Input: part model. Units: mm. Frame: model coordinates. A direction names the side the tool comes from. Coordinates: 2 decimals unless noted, no trailing zeros. Write each loop counter-clockwise with the first axis right and the second up, starting at its lowest first coordinate (ties: lowest second). Pieces come first, ordered by that corner, then holes. Notation, with made-up numbers: M 57.25,89 L 109.25,89 A20 cw 109.25,110 Z; hole C -33.5,56.25 d5. An arc over 180 degrees is marked long. Use CSV: the item, a comma, the result in double quotes.
Autodesk Inventor part; units mm, degrees
ref_plane "YZ Plane" through (0, 0, 0) normal (1, 0, 0) x (0, 1, 0)
ref_plane "XZ Plane" through (0, 0, 0) normal (0, 1, 0) x (-1, 0, 0)
ref_plane "XY Plane" through (0, 0, 0) normal (0, 0, 1) x (1, 0, 0)
sketch "Sketch1" plane through (0, 0, 0) normal (0, 1, 0) x (-1, 0, 0)
  circle A0 centre (0, 0) radius 10 construction
  circle A1 centre (0, 0) radius 16
  circle A2 centre (0, 0) radius 11
  circle A3 centre (0, 0) radius 9
  dimension "d0" = 20
  dimension "d1" = 6
  dimension "d4" = 1
  dimension "d9" = 2
extrude "Extrusion1" add sketch "Sketch1" along normal blind 2 contours A1 | A2 | A3
extrude "Extrusion2" add sketch "Sketch1" against normal blind 3 contours A2 | A3
extrude "Extrusion4" cut sketch "Sketch1" along normal through all both and the other way through all contours A3
sketch "Sketch4" plane through (0, 2, 0) normal (0, 1, 0) x (1, 0, 0)
  circle A0 centre (0, 0) radius 16
  line L0 (16, -14.5) -> (-16, -14.5)
  line L1 (-16, -14.5) -> (-16, 14.5)
  line L2 (-16, 14.5) -> (16, 14.5)
  line L3 (16, 14.5) -> (16, -14.5)
  line L4 (16, -14.5) -> (-16, 14.5) construction
  line L5 (-16, -14.5) -> (16, 14.5) construction
  line L6 (-17.5, -16) -> (17.5, -16)
  line L7 (17.5, -16) -> (17.5, 16)
  line L8 (17.5, 16) -> (-17.5, 16)
  line L9 (-17.5, 16) -> (-17.5, -16)
  dimension "d18" = 29
extrude "Extrusion6" cut sketch "Sketch4" against normal up to surface (2 mm away) contours L3 L2 A0 L8 L7 L6 L0 | L2 A0 | A0 L0 | A0 L2 L1 L0 L6 L9 L8
fillet "Fillet1" radius 5 4 edges at (-6.7639, 1, 14.5) (6.7639, 1, 14.5) (-6.7639, 1, -14.5) (6.7639, 1, -14.5)
fillet "Fillet2" radius 1 8 edges at (-6.8509, 0, 14.3265) (6.8509, 0, 14.3265) (0, 0, 14.5) (-16, 0, 0) (16, 0, 0) (-6.8509, 0, -14.3265) (6.8509, 0, -14.3265) (0, 0, -14.5)
equation "\"d0\" = FilterDia"
equation "\"MaskHeight\" = 125"
equation "\"FilterDia\" = 20"
equation "\"NoseWidth\" = 25"
equation "\"MaterialThickness\" = 2"
equation "\"Tol\" = 0.25"
equation "\"MaterialHardness\" = 0.3"
equation "\"ClipHeight\" = 4"
equation "\"ClipWidth\" = 5"
equation "\"ClipNeck\" = 5"
equation "\"ValveNeckDia\" = 3"
equation "\"ValveNeckLength\" = 2"
equation "\"ValveFlapDia\" = 19.25"
equation "\"LeftValve\" = 0"
equation "\"RightValve\" = 0"
equation "\"CoreScrewHeadDia\" = 9.525"
equation "\"CoreScrewLength\" = 50.8"
equation "\"CoreScrewID\" = 2.38125"
equation "\"CoreScrewOD\" = 3.96875"
equation "\"StrapAttachmentNeckDia\" = 6.5"
equation "\"StrapAttachmentNeckHeight\" = 1.5"
equation "\"StrapNoseRadialDifference\" = 2"
equation "\"StrapNoseHeight\" = 7.5"
equation "\"ZipTieThickness\" = 4"
equation "\"PinTol\" = 0.75"
equation "\"PinDia\" = 7"
equation "\"PinDepth\" = 5"
properties part number "FilterPort_Printable"
1. Material intervals for line 1 (Z direction, x = 0, y = 0.95); line 2 (Z direction, x = 0, y = -1.95); line 3 (X direction, y = -2.7, z = -8.25), sorted ascending. Write a range as [from, to].
Resolved:
line 1,"z = [-14.5, -9], [9, 14.5]"
line 2,"z = [-11, -9], [9, 11]"
line 3,"x = [-7.28, -3.6], [3.6, 7.28]"
2. Access query for faces 1 (the flat face through (7, 0, 9)), 2 (the cylindrical face through (16, 1.5, -0.2)). Directions: +Z, -Z, +X, -X, +Y, -Y. A direction counts if a zero-diameter tool reaches every point of the face in a straight line with its end or side. Return the directions, or none.
Resolved:
face 1,"-Y"
face 2,"+X, +Y, -Y"
3. Section B-B (x = 0). Return loops of the section in (y, z).
Resolved:
outline,"M -3,-11 L 0,-11 L 0,-13.5 A1 ccw 1,-14.5 L 2,-14.5 L 2,-9 L -3,-9 Z; M -3,9 L 2,9 L 2,14.5 L 1,14.5 A1 ccw 0,13.5 L 0,11 L -3,11 Z"
4. Section C-C (y = 1.4). Return loops of the section in (x, z), then the cut area to 3 significant figures.
Resolved:
outline,"M -8.07,-13.82 A5 ccw -5.55,-14.5 L 5.55,-14.5 A5 ccw 8.07,-13.82 A16 ccw 8.07,13.82 A5 ccw 5.55,14.5 L -5.55,14.5 A5 ccw -8.07,13.82 A16 ccw Z; hole C 0,0 d18"
area,"522 mm^2"
5. Section D-D (y = -0.45). Return loops of the section in (x, z), then the cut area to 3 significant figures.
Resolved:
outline,"C 0,0 d22; hole C 0,0 d18"
area,"126 mm^2"
6. Mould query, pull axis X, two halves, no side actions, for faces 3 (the cylindrical face through (1.172, -0.535, -8.923)), 4 (the flat face through (-2, -3, -9)), 5 (the cylindrical face through (-6.87, 1.49, -14.32)). Classes: pulls with the +X half, pulls with the -X half, needs draft (parallel to the pull), parting line crosses it, or undercut.
Resolved:
face 3,"undercut"
face 4,"needs draft"
face 5,"pulls with the -X half"
7. Section A-A (z = 0). Return loops of the section in (x, y).
Resolved:
outline,"M -16,1 A1 ccw -15,0 L -11,0 L -11,-3 L -9,-3 L -9,2 L -16,2 Z; M 9,-3 L 11,-3 L 11,0 L 15,0 A1 ccw 16,1 L 16,2 L 9,2 Z"
8. Contact query for a flat-ended pin moving along its axis: pin 1 Ø14.5 at (x, z) = (0, 0) entering from -Y. Output: stop coordinate, or through.
Resolved:
pin 1,"passes through"
